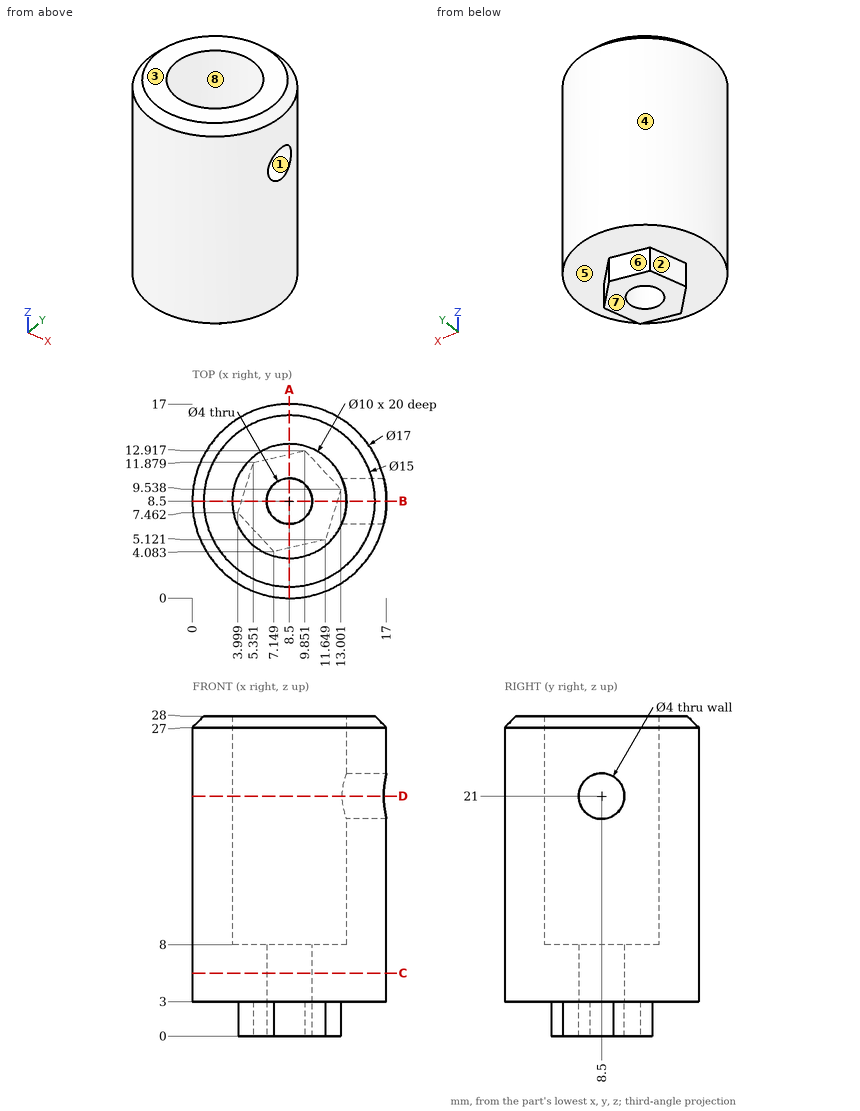
Print and shaded views of the part. All mm, measured from the part's lowest x, y and z. A direction names the side the tool comes from. Round coordinates to 2 decimals unless told otherwise and drop trailing zeros. Write each loop counter-clockwise with the first axis right and the second up, starting at its lowest first coordinate (ties: lowest second). Pieces come first, ordered by that corner, then holes. Notation, with made-up numbers: M -10,84.25 L 6,84.25 A28 cw 6,103.25 Z; hole C -38,77 d6. An arc over 180 degrees is marked long. Use a Markdown table: item, result. Add a question column.
1. Slice it at B-B on y = 8.5. Give the cut face in (x, z).
2. Pull direction Z, two halves, no side cores. Call the marked faces 1, 2 and 3: released by +Z, released by -Z, zero draft, split by the parting line, or undercut.
3. Slice it at C-C on z = 5.5. Give the cut face in (x, y).
4. Drill centre lines: probe 1 along Y at (x, z) = (8.5, 24); probe 2 along Y at (x, z) = (8.5, 6.4); probe 3 along Z at (x, y) = (2.25, 9.5). Where is each one in solid material? Low to high.
5. Flat gauge pins, fed straight in: P1, Ø2.5, axis at y = 8.5, z = 21, coming from the +X side; P2, Ø3, axis at y = 10.5, z = 24.5, coming from the -X side (1 decimal); P3, Ø3, axis at y = 14, z = 22, coming from the +X side. Where does each tip first touch, or does it go through?
6. Slice it at A-A on x = 8.5. Give the cut face in (y, z) (1 decimal).
7. 3-axis set-ups, long thin cutter, end or side, ignore diameter. For the marked faces 4, 5, 6, 7 and 8: which of +Z, -Z, +X, -X, +Y, -Y reach the whole face in a straight line?
8. Slice it at D-D on z = 21. Give the cut face in (x, y), then the cut area to 3 significant figures.
Reply:
| question | item | result |
|---|---|---|
| 1 | outline | M 0,3 L 4.32,3 L 4.32,0 L 6.5,0 L 6.5,8 L 3.5,8 L 3.5,28 L 1,28 L 0,27 Z; M 10.5,0 L 12.68,0 L 12.68,3 L 17,3 L 17,19 L 13.5,19 L 13.5,8 L 10.5,8 Z; M 13.5,23 L 17,23 L 17,27 L 16,28 L 13.5,28 Z |
| 2 | face 1 | undercut |
| 2 | face 2 | zero draft |
| 2 | face 3 | released by +Z |
| 3 | outline | C 8.5,8.5 d17; hole C 8.5,8.5 d4 |
| 4 | probe 1 | y = 0 to 3.5, 13.5 to 17 |
| 4 | probe 2 | y = 0 to 6.5, 10.5 to 17 |
| 4 | probe 3 | z = 3 to 28 |
| 5 | P1 | stops at x = 3.66 |
| 5 | P2 | stops at x = 0 |
| 5 | P3 | stops at x = 16 |
| 6 | outline | M 0,3 L 4.4,3 L 4.4,0 L 6.5,0 L 6.5,8 L 3.5,8 L 3.5,28 L 1,28 L 0,27 Z; M 10.5,0 L 12.6,0 L 12.6,3 L 17,3 L 17,27 L 16,28 L 13.5,28 L 13.5,8 L 10.5,8 Z |
| 7 | face 4 | +Z, -Z |
| 7 | face 5 | -Z |
| 7 | face 6 | -Z, -X, +Y |
| 7 | face 7 | -Z, +X, -X, +Y, -Y |
| 7 | face 8 | +Z |
| 8 | outline | M 13.08,6.5 A5 cw long 13.08,10.5 L 16.76,10.5 A8.5 ccw long 16.76,6.5 Z |
| 8 | area | 134 mm^2 |
